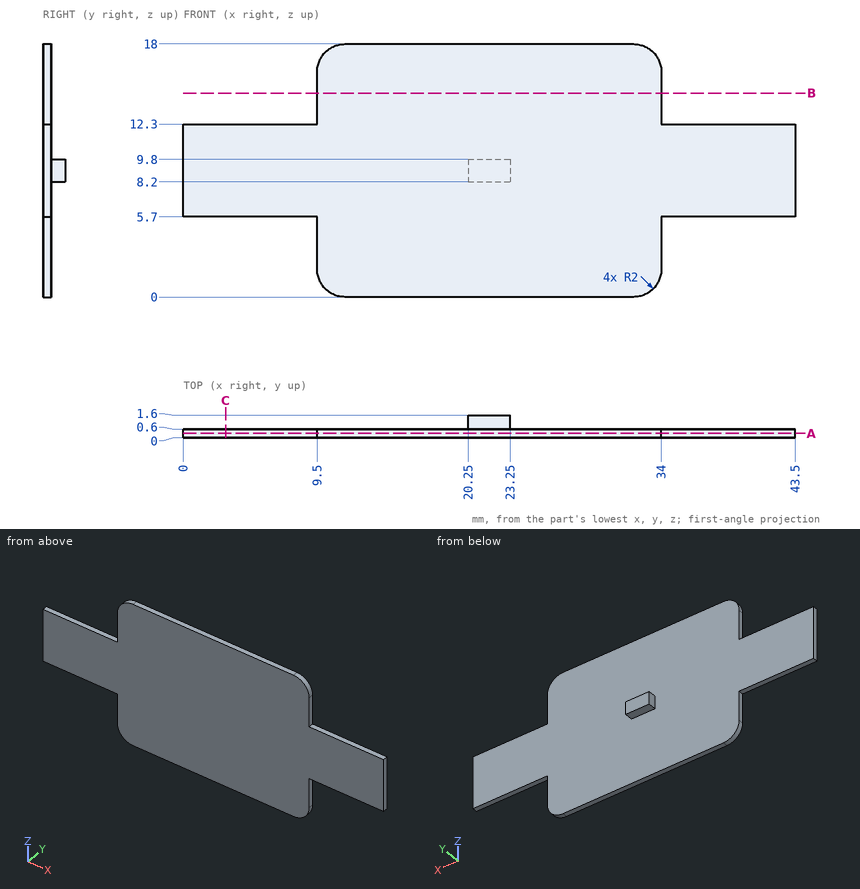
Source: three-view drawing plus pictorial views. Frame: mm from the lowest corner of the part. Round coordinates to 2 decimals unless told otherwise and drop trailing zeros. Loops run counter-clockwise (first coordinate to the right, second up) from the corner with the lowest first, then second, coordinate; pieces in that order, holes last. Notation, with made-up numbers: M -8.5,6.25 L 6.5,6.25 A29 cw 6.5,37.25 Z; hole C 60,-35.5 d4. An arc over 180 degrees is marked long. Put each result on its own line as item: value. Start each with the question number.
(1) Section query B-B (z = 14.5). Return loops of the section in (x, y), then the cut area to 3 significant figures.
(2) Material intervals for line 1 along Y through (x, z) = (5.5, 12.25); line 2 along X through (y, z) = (1.5, 8.75); line 3 along X through (y, z) = (0.55, 3.75), sorted ascending. Write a range as [from, to].
(3) Contact query for flat-ended pins moving along their axis: pin 1 Ø0.7 at (x, y) = (36.5, 0) entering from -Z; pin 2 Ø0.8 at (x, y) = (21.5, 1.5) entering from -Z; pin 3 Ø0.5 at (y, z) = (0.5, 3.5) entering from -X; pin 4 Ø1 at (x, z) = (7, 13) entering from -Y. Output: stop coordinate, or through.
(4) Section query A-A (y = 0.3). Return loops of the section in (x, z), then the cut area to 3 significant figures.
(5) Section query C-C (x = 3). Return loops of the section in (y, z).
Findings below:
1. outline: M 9.5,0 L 34,0 L 34,0.6 L 9.5,0.6 Z
1. area: 14.7 mm2
2. line 1: y = [0, 0.6]
2. line 2: x = [20.25, 23.25]
2. line 3: x = [9.5, 34]
3. pin 1: stops at z = 5.7
3. pin 2: stops at z = 8.2
3. pin 3: stops at x = 9.5
3. pin 4: passes through
4. outline: M 0,5.7 L 9.5,5.7 L 9.5,2 A2 ccw 11.5,0 L 32,0 A2 ccw 34,2 L 34,5.7 L 43.5,5.7 L 43.5,12.3 L 34,12.3 L 34,16 A2 ccw 32,18 L 11.5,18 A2 ccw 9.5,16 L 9.5,12.3 L 0,12.3 Z
4. area: 563 mm2
5. outline: M 0,5.7 L 0.6,5.7 L 0.6,12.3 L 0,12.3 Z
